Autodesk Inventor part; units mm, degrees
ref_plane "Arbeitsebene1" through (0, 0, 0) normal (1, 0, 0) x (0, 0, -1)
ref_plane "YZ Plane" through (0, 0, 0) normal (1, 0, 0) x (0, 1, 0)
ref_plane "XZ Plane" through (0, 0, 0) normal (0, 1, 0) x (-1, 0, 0)
ref_plane "Arbeitsebene1" through (0, 0, 0) normal (1, 0, 0) x (0, 0, -1)
sketch "Skizze1" plane through (0, 0, 0) normal (1, 0, 0) x (0, 0, -1)
  arc A0 (14.55, 0) -> (-14.55, 0) centre (0, 0) ccw
  circle A1 centre (0, 0) radius 5.5
  line L0 (-20.8128, 0) -> (22.3238, 0) construction
  line L1 (0, -22.3037) -> (0, 20.6923) construction
  circle A2 centre (0, 10.45) radius 1
  circle A3 centre (-9.05, -5.225) radius 1
  circle A4 centre (9.05, -5.225) radius 1
  circle A5 centre (0, 0) radius 10.45 construction
  line L2 (0, 0) -> (9.05, -5.225) construction
  line L3 (0, 0) -> (-9.05, -5.225) construction
  line L4 (8.89, -5.5) -> (-8.89, -5.5) construction
  line L5 (-8.89, -5.5) -> (-8.89, 5.5) construction
  line L6 (-8.89, 5.5) -> (8.89, 5.5) construction
  line L7 (8.89, 5.5) -> (8.89, -5.5) construction
  circle A6 centre (8.89, 5.5) radius 1.2
  circle A7 centre (-8.89, 5.5) radius 1.2
  arc A8 (-14.55, 0) -> (14.1469, 3.4013) centre (0, 0) ccw
  line L8 (8.89, 7.7) -> (-8.89, 7.7)
  line L9 (6.5, 3.3) -> (6.5, 7.7)
  line L10 (-4.3414, 8.5633) -> (-4.3414, 8.4781)
  line L11 (-6.5, 7.7) -> (-6.5, 3.3)
  arc A9 (4.4, 3.3) -> (-4.4, 3.3) centre (0, 0) ccw
  line L12 (6.5, 3.3) -> (4.4, 3.3)
  line L13 (-4.4, 3.3) -> (-6.5, 3.3)
  line L14 (-6.5, -13.0174) -> (-6.5, -7.45)
  line L15 (6.5, -13.0174) -> (6.5, -7.45)
  line L16 (11.09, -9.4188) -> (11.09, -7.45)
  circle A10 centre (8.89, -5.5) radius 1.2
  circle A11 centre (-8.89, -5.5) radius 1.2
  line L17 (11.09, -7.45) -> (11.09, 5.5)
  line L18 (-6.5, -7.45) -> (-6.5, 3.3)
  line L19 (-11.09, -7.45) -> (-11.09, 5.5)
  arc A12 (-8.89, 7.7) -> (-11.09, 5.5) centre (-8.89, 5.5) ccw
  arc A13 (11.09, 5.5) -> (8.89, 7.7) centre (8.89, 5.5) ccw
  arc A14 (7.7675, -7.45) -> (10.0125, -7.45) centre (8.89, -5.5) ccw
  line L20 (6.5, -7.45) -> (7.7675, -7.45)
  line L21 (10.0125, -7.45) -> (11.09, -7.45)
  arc A15 (-10.0125, -7.45) -> (-7.7675, -7.45) centre (-8.89, -5.5) ccw
  line L22 (-11.09, -7.45) -> (-10.0125, -7.45)
  line L23 (-7.7675, -7.45) -> (-6.5, -7.45)
  line L24 (6.5, -7.45) -> (6.5, 3.3)
  line L25 (-11.09, -7.45) -> (-11.09, -9.4188)
  point P0 (0, 14.55)
  dimension "d2" = 11
  dimension "d9" = 2
  dimension "d11" = 120
  dimension "d12" = 20.9
  dimension "d19" = 11
  dimension "d20" = 17.78
  dimension "d22" = 2.4
  dimension "d29" = 14.55
  dimension "d30" = 5.5
  dimension "d38" = 2.2
  dimension "d39" = 13
  dimension "d42" = 4.5
  dimension "d43" = 0.3
extrude "Extrusion1" add sketch "Skizze1" against normal blind 2 contours A8 L16 L17 A13 L8 A12 L19 L25 A0 | A8 L15 L20 A14 L21 L16 | A8 L14 L18 L13 A1 L12 L24 L15 | L21 A14 L20 L24 L9 L8 A13 L17 | L25 L22 A15 L23 L14 A8 | L19 A12 L8 L11 L18 L23 A15 L22 | L12 A1 L13 L11 L8 L9 | A3 A11 | A4 A10 | A6 | A7 picked at (-8.3922, -6.3901) picked at (8.4037, -6.3962)
extrude "Extrusion3" add sketch "Skizze1" against normal blind 13.2 from surface at -2 contours A8 L15 L20 A14 L21 L16 | L25 L22 A15 L23 L14 A8 | L12 A1 L13 L11 L8 L9
extrude "Extrusion4" add sketch "Skizze1" against normal blind 3 from surface at -15.2 contours A8 L15 L20 A14 L21 L16 | L21 A14 L20 L24 L9 L8 A13 L17 | L25 L22 A15 L23 L14 A8 | L19 A12 L8 L11 L18 L23 A15 L22 | L12 A1 L13 L11 L8 L9 | A11 A3 | A10 A4 picked at (-9.542, -4.4536) picked at (9.542, -4.4536)
properties part number "AS5047DEnclosure"
Here's how the part is built. I have some questions about the finished solid (model axes, mm). A direction names the side the tool comes from. Round coordinates to 2 decimals unless told otherwise and drop trailing zeros. Order: outer loops, then holes, each group sorted by start corner. A loop starts at its lowest first (then second) coordinate and runs counter-clockwise, first axis right, second up. Notation, with made-up numbers: M -21,66.5 L 14,66.5 A29 cw 14,102.5 Z; hole C 72.5,-19 d8. An arc over 180 degrees is marked long. Answer in a Markdown table with one row per item.
Item 1: Imagine slicing it at B-B, the plane z = -3.5. Write out the boundary of the cut face in (x, y), and give its area (3 significant figures).
A:
| item | result |
|---|---|
| outline | M -18.2,4.24 L 0,4.24 L 0,14.12 L -2,14.12 L -2,7.7 L -18.2,7.7 Z; M -2,-14.12 L 0,-14.12 L 0,-4.24 L -2,-4.24 Z |
| area | 95.5 mm2 |
Item 2: If I drill on L1, parallel to Z at x = -17.5, y = -5.5; L2, parallel to X at y = 1.25, z = 7; L3, parallel to Y at x = -16.8, z = -8.89, over which ranges is the centre line in solid material (lowest first)? Write a range as from..to.
A:
| item | result |
|---|---|
| L1 | z = -11.09..-10.09, -7.69..-6.5, 6.5..7.69, 10.09..11.09 |
| L2 | x = -18.2..-15.2, -2..0 |
| L3 | y = -11.52..-6.7, -4.3..4.3, 6.7..7.7 |
Item 3: I'm going to push flat-ended pins straight in: pin 1 (5 mm diameter, centred on x = -7.5, y = -6.5, fed in from -Z); pin 2 (10 mm diameter, centred on y = 0, z = 0, fed in from -X); pin 3 (3 mm diameter, centred on x = -9, z = 4, fed in from -Y); pin 4 (1 mm diameter, centred on x = -14.5, z = 6, fed in from +Y). Where does each tip first touch, or does it pass through?
A:
| item | result |
|---|---|
| pin 1 | stops at z = -11.09 |
| pin 2 | passes through |
| pin 3 | stops at y = 3.3 |
| pin 4 | stops at y = 7.7 |
Item 4: Imagine slicing it at C-C, the plane z = 0. Write out the boundary of the cut face in (x, y), and give its area (3 significant figures).
A:
| item | result |
|---|---|
| outline | M -18.2,5.5 L 0,5.5 L 0,9.45 L -2,9.45 L -2,7.7 L -18.2,7.7 Z; M -2,-14.55 L 0,-14.55 L 0,-5.5 L -2,-5.5 Z; M -2,11.45 L 0,11.45 L 0,14.55 L -2,14.55 Z |
| area | 67.8 mm2 |
Item 5: Imagine slicing it at A-A, the plane y = 10.45. Write out the boundary of the cut face in (x, z).
A:
| item | result |
|---|---|
| outline | M -2,-10.12 L 0,-10.12 L 0,-1 L -2,-1 Z; M -2,1 L 0,1 L 0,10.12 L -2,10.12 Z |
Item 6: Imagine slicing it at D-D, the plane y = 0.75. Write out the boundary of the cut face in (x, z).
A:
| item | result |
|---|---|
| outline | M -18.2,-11.09 L -15.2,-11.09 L -15.2,-6.5 L -18.2,-6.5 Z; M -18.2,6.5 L -15.2,6.5 L -15.2,11.09 L -18.2,11.09 Z; M -2,-14.53 L 0,-14.53 L 0,-5.45 L -2,-5.45 Z; M -2,5.45 L 0,5.45 L 0,14.53 L -2,14.53 Z |
Item 7: Thinking about a two-plate mould opening in Z: for faces 1 (the face through (-16.679, 6.311, 9.774)), 2 (the face through (-0.97, -14.44, 1.8)), 3 (the face through (-12, -9, 6.5)), 4 (the face through (-9, -7.45, 7)), which applies, +Z half, -Z half, draft (parallel to the pull), parting line (faces both ways), or undercut?
A:
| item | result |
|---|---|
| face 1 | undercut |
| face 2 | parting line |
| face 3 | undercut |
| face 4 | draft |
Item 8: For faces 5 (the face through (-12, -9, -6.5)), 6 (the face through (-2, 0, -6)), 7 (the face through (-9, -7.45, -7)), which set-ups out of +Z, -Z, +X, -X, +Y, -Y let a thin tool reach every point of the face, with its end or its side?
A:
| item | result |
|---|---|
| face 5 | -X, -Y |
| face 6 | none |
| face 7 | +Z, -Z, +Y |
